Input: dimensioned drawing with shaded views. Units: mm. Origin: part minimum x, y, z. A direction names the side the tool comes from. Give positions to 0.01 mm unless a question says otherwise; leave off trailing zeros. Write each loop counter-clockwise with the first axis right and the second up, starting at its lowest first coordinate (ties: lowest second). Pieces come first, ordered by that corner, then holes. Notation, with made-up numbers: (7, 20) -> (51, 20) arc R16 ccw to (51, 37) -> close; hole circle Ø9 at (42.25, -29.75). An arc over 180 degrees is marked (long way). Answer as a JSON object with one key per item and string values. Group by question number.
(1) Section query D-D on x = 5.5. Output: boundary loops of the cut face in (y, z).
(2) Material intervals for probe 1 along X at (y, z) = (15, 3); probe 2 along X at (y, z) = (4.75, 4.25); probe 3 along Y at (x, z) = (15.8, 3.75), sorted ascending.
(3) Section query A-A on y = 6. Output: boundary loops of the cut face in (x, z), plus the area to 3 significant figures.
(4) Draft query along X for the marked faces 4, 5 and 6. Return one class per face: +X half, -X half, draft (parallel to the pull), parting line (faces both ways), or undercut.
(5) Contact query for a flat-ended pin moving along its axis: pin 1 Ø0.5 at (x, z) = (2.5, 4) entering from +Y. Output: stop coordinate, or through.
(6) Set-up query: the marked faces 1, 2 and 3. Return all of +Z, -Z, +X, -X, +Y, -Y with unobstructed straight access to the full face (end or side cutting, diameter ignored); none if empty.
(7) Section query C-C on z = 0.5. Output: boundary loops of the cut face in (x, y).
(8) Section query B-B on x = 21.5. Output: boundary loops of the cut face in (y, z), plus the area to 3 significant figures.
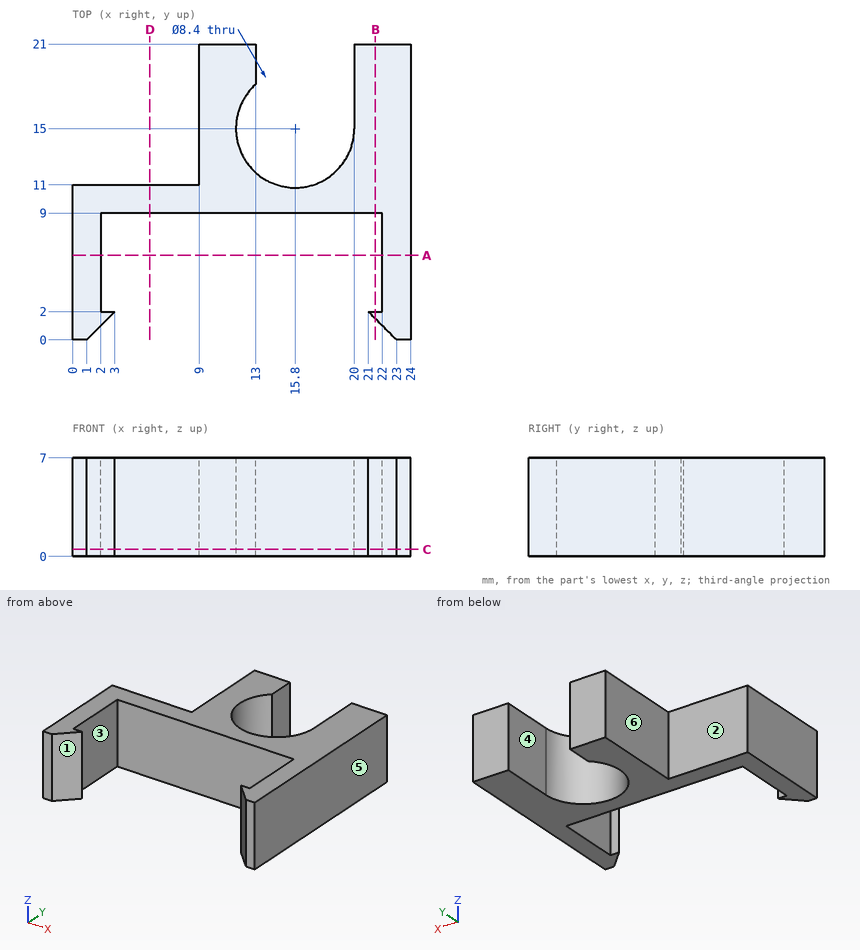
Answer list:
{
 "1": {"outline": "(9, 0) -> (11, 0) -> (11, 7) -> (9, 7) -> close"},
 "2": {"probe 1": "9 to 11.6, 20 to 24", "probe 2": "0 to 2, 22 to 24", "probe 3": "9 to 10.8"},
 "3": {"outline": "(0, 0) -> (2, 0) -> (2, 7) -> (0, 7) -> close; (22, 0) -> (24, 0) -> (24, 7) -> (22, 7) -> close", "area": "28.0 mm2"},
 "4": {"face 4": "undercut", "face 5": "+X half", "face 6": "-X half"},
 "5": {"pin 1": "y = 11"},
 "6": {"face 1": "+Z, -Z, -Y", "face 2": "+Z, -Z, -X, +Y", "face 3": "+Z, -Z"},
 "7": {"outline": "(0, 0) -> (1, 0) -> (3, 2) -> (2, 2) -> (2, 9) -> (22, 9) -> (22, 2) -> (21, 2) -> (23, 0) -> (24, 0) -> (24, 21) -> (20, 21) -> (20, 15) arc R4.2 cw (long way) to (13, 18.13) -> (13, 21) -> (9, 21) -> (9, 11) -> (0, 11) -> close"},
 "8": {"outline": "(1.5, 0) -> (2, 0) -> (2, 7) -> (1.5, 7) -> close; (9, 0) -> (21, 0) -> (21, 7) -> (9, 7) -> close", "area": "87.5 mm2"}
}
